Verification items for the finished model (mm, model axes). Round coordinates to 2 decimals unless told otherwise and drop trailing zeros. Write each loop counter-clockwise with the first axis right and the second up, starting at its lowest first coordinate (ties: lowest second). Pieces come first, ordered by that corner, then holes. Notation, with made-up numbers: M 75.25,85.5 L 91.25,85.5 A23 ccw 91.25,95.5 Z; hole C 10.25,45.5 d10. An arc over 180 degrees is marked long. Use a Markdown table: item, result. Add a question column.
from build123d import *

# Parameters (mm, degrees)
BOSS_EXTRUDE1_DEPTH = 10
SKETCH2_R           = 16.25
BOSS_EXTRUDE2_DEPTH = 10
SKETCH3_R           = 16.25
CUT_EXTRUDE1_DEPTH  = 10


with BuildPart() as part:
    # Sketch1 → Boss-Extrude1 (new body)
    with BuildSketch(Plane.XY):
        with BuildLine():
            ThreePointArc((-125, 25), (-150, 0), (-125, -25))
            ThreePointArc((-125, -25), (0, -14.509972887), (125, -25))
            ThreePointArc((125, -25), (150, 0), (125, 25))
            ThreePointArc((125, 25), (0, 14.509972887), (-125, 25))
        make_face()
    extrude(amount=BOSS_EXTRUDE1_DEPTH)

    # Sketch2 → Boss-Extrude2 (add)
    with BuildSketch(Plane(origin=(0, 0, 0), x_dir=(1, 0, 0), z_dir=(0, 0, -1))):
        with Locations((-125, 0)):
            Circle(SKETCH2_R)
    extrude(amount=BOSS_EXTRUDE2_DEPTH)

    # Sketch3 → Cut-Extrude1 (cut)
    with BuildSketch(Plane.XY.offset(10)):
        with Locations((125, 0)):
            Circle(SKETCH3_R)
    extrude(amount=-CUT_EXTRUDE1_DEPTH, mode=Mode.SUBTRACT)


solid = part.part
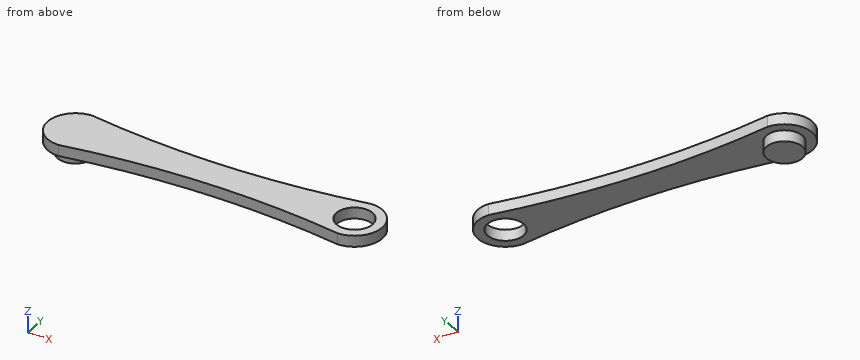
1. Cross-section at C-C on y = 19. Enter the section's corners in (x, z).
2. Scan lines: line 1 along Y through (x, z) = (125, 3.5); line 2 along X through (y, z) = (1, 7.75); line 3 along X through (y, z) = (-0.5, -8.25). Record each from-to range of solid material in increasing order. Write a range as from..to.
3. Depth check by flat-ended pin: pin 1 Ø6 at (x, y) = (52, 19) entering from -Z; pin 2 Ø4 at (y, z) = (-14, 7) entering from -X. Enter the tip coordinate at first touch or a pass-through.
4. Cross-section at B-B on z = 3.25. Enter the section's corners in (x, y), plus the area to 3 significant figures.
5. Cross-section at A-A on y = 0. Enter the section's corners in (x, z), plus the area to 3 significant figures.
6. Cross-section at D-D on x = -60.5. Enter the section's corners in (y, z).
Answer:
| question | item | result |
|---|---|---|
| 1 | outline | M -141.25,0 L -81.94,0 L -81.94,10 L -141.25,10 Z; M 81.94,0 L 141.25,0 L 141.25,10 L 81.94,10 Z |
| 2 | line 1 | y = -25..-16.25, 16.25..25 |
| 2 | line 2 | x = -149.98..108.78, 141.22..149.98 |
| 2 | line 3 | x = -141.24..-108.76 |
| 3 | pin 1 | stops at z = 0 |
| 3 | pin 2 | stops at x = -146.93 |
| 4 | outline | M -125,-25 A750 cw 125,-25 A25 ccw 125,25 A750 cw -125,25 A25 ccw Z; hole C 125,0 d32.5 |
| 4 | area | 10,100 mm^2 |
| 5 | outline | M -150,0 L -141.25,0 L -141.25,-10 L -108.75,-10 L -108.75,0 L 108.75,0 L 108.75,10 L -150,10 Z; M 141.25,0 L 150,0 L 150,10 L 141.25,10 Z |
| 5 | area | 3,000 mm^2 |
| 6 | outline | M -16.95,0 L 16.95,0 L 16.95,10 L -16.95,10 Z |
